Autodesk Inventor part; units mm, degrees
ref_plane "РабПлоскость7" through (-34.5, 0, 0) normal (-1, 0, 0) x (0, 0, 1)
ref_plane "YZ Plane" through (0, 0, 0) normal (1, 0, 0) x (0, 1, 0)
ref_plane "XZ Plane" through (0, 0, 0) normal (0, 1, 0) x (-1, 0, 0)
sketch "Эскиз1" plane through (0, 0, 0) normal (0, 1, 0) x (-1, 0, 0)
  line L0 (0, 0) -> (69, 0)
  line L1 (69, 0) -> (69, -52)
  line L2 (69, -52) -> (0, -52)
  line L3 (0, -52) -> (0, 0)
  line L4 (0, -26) -> (32, -26)
  line L5 (64, -10) -> (0, -10)
  line L6 (0, -10) -> (0, -42)
  line L7 (0, -42) -> (64, -42)
  line L8 (64, -42) -> (64, -10)
  line L9 (64, -10) -> (0, -42) construction
  line L10 (0, -10) -> (64, -42) construction
  line L11 (0, -10) -> (2, -10)
  point P0 (0, -10)
  dimension "d0" = 69
  dimension "d224" = 10
  dimension "d225" = 5
  dimension "d226" = 32
extrude "Выдавливание1" add sketch "Эскиз1" along normal blind 15 contours L0 L1 L2 L3 L7 L8 L5
sketch "Эскиз2" plane through (0, 15, 0) normal (0, 1, 0) x (1, 0, 0)
  line L0 (-8.5, 3.5) -> (-60.5, 3.5)
  line L1 (-60.5, 3.5) -> (-60.5, 48.5)
  line L2 (-60.5, 48.5) -> (-8.5, 48.5)
  line L3 (-8.5, 48.5) -> (-8.5, 3.5)
  line L4 (-8.5, 3.5) -> (-60.5, 48.5) construction
  line L5 (-60.5, 3.5) -> (-8.5, 48.5) construction
  line L6 (0, 0) -> (0, 10)
  line L7 (-69, 52) -> (-69, 0)
  line L8 (0, 52) -> (-69, 52) construction
  line L9 (0, 10) -> (0, 42) construction
  line L10 (-69, 26) -> (0, 26) construction
  point P0 (-34.5, 26)
  point P1 (-34.5, 26)
  point P2 (-60.5, 26)
  point P3 (-34.5, 26)
  dimension "d227" = 52
  dimension "d228" = 45
extrude "Выдавливание2" cut sketch "Эскиз2" against normal blind 3.5
sketch "Эскиз3" plane through (0, 11.5, 0) normal (0, 1, 0) x (1, 0, 0)
  circle A0 centre (-57.5, 45.5) radius 3
  circle A1 centre (-11.5, 45.5) radius 3
  line L0 (-60.5, 48.5) -> (-8.5, 48.5)
  line L1 (-8.5, 48.5) -> (-8.5, 42)
  line L2 (-8.5, 42) -> (-60.5, 42)
  line L3 (-60.5, 42) -> (-60.5, 48.5)
  line L4 (-60.5, 10) -> (-8.5, 10)
  line L5 (-8.5, 42) -> (-60.5, 42)
  line L6 (-8.5, 48.5) -> (-8.5, 42)
  line L7 (-60.5, 48.5) -> (-8.5, 48.5)
  line L8 (-60.5, 42) -> (-60.5, 48.5)
  line L9 (-60.5, 3.5) -> (-60.5, 10)
  line L10 (-8.5, 3.5) -> (-60.5, 3.5)
  line L11 (-8.5, 10) -> (-8.5, 3.5)
  line L12 (0, 10) -> (-64, 10)
  line L13 (-8.5, 3.5) -> (-60.5, 3.5)
  line L14 (-32, 3.5) -> (-37, 3.5)
  line L15 (-37, 3.5) -> (-37, 5.5)
  line L16 (-37, 5.5) -> (-32, 5.5)
  line L17 (-32, 5.5) -> (-32, 3.5)
  line L18 (-8.5, 3.5) -> (-60.5, 3.5)
  point P0 (-38, 39.1)
  point P1 (-60.5, 45.5)
  point P2 (-8.3, 39.1)
  point P3 (-5.8, 45.225)
  point P4 (-57.5, 48.5)
  point P5 (-11.5, 48.5)
  point P6 (-8.5, 42.24)
  point P7 (-8.5, 45.5)
  point P8 (-34.5, 3.5)
  dimension "d236" = 3
  dimension "d237" = 3
  dimension "d238" = 3
  dimension "d239" = 3
  dimension "d240" = 6
  dimension "d241" = 6
  dimension "d304" = 2
  dimension "d305" = 5
extrude "Выдавливание5" add sketch "Эскиз3" along normal blind 3 contours A0 | A0 L3 L0 | L0 L1 A1 | A1 | L15 L16 L17 L10
sketch "Эскиз4" plane through (-71.3, 14.5, -19.65) normal (0, 1, 0) x (0, 0, -1)
  arc A0 (25.85, -10.8) -> (28.85, -13.8) centre (25.85, -13.8) ccw
  arc A1 (28.85, -59.8) -> (25.85, -62.8) centre (25.85, -59.8) ccw
hole "Отверстие1" at (-57.5, 14.5, -45.5) at (-11.5, 14.5, -45.5) direction (0, -1, 0) diameter 3 depth 5
sketch "Эскиз32" plane through (0, 11.5, 0) normal (0, 1, 0) x (1, 0, 0)
  line L0 (-64, 10) -> (-64, 42)
  line L1 (-64, 47.775) -> (-43.5, 47.775)
  line L2 (-8.5, 3.5) -> (-60.5, 3.5)
  line L3 (-8.5, 10) -> (-8.5, 3.5)
  line L4 (-60.5, 48.5) -> (-8.5, 48.5)
  line L5 (-8.5, 48.5) -> (-8.5, 42)
  point P0 (0, 0)
  point P1 (-17.6, 6.862)
  point P2 (-5.3, 5.3)
  point P3 (-8.3, 2.3)
  point P4 (-64, 4.225)
  point P5 (-17.6, 45.087)
  dimension "d261" = 3.362
  dimension "d263" = 9.1
  dimension "d296" = 3.413
  dimension "d297" = 9.1
hole "Отверстие5" at (-17.6, 11.5, -6.862) at (-17.6, 11.5, -45.087) direction (0, -1, 0) diameter 3.2 end through all countersink diameter 6 countersink angle 90
sketch "Эскиз12" plane through (0, 15, 0) normal (0, -1, 0) x (1, 0, 0)
  line L0 (-60.5, -48.5) -> (-8.5, -48.5)
  line L1 (0, -52) -> (-69, -52)
  line L2 (-35.9, -52) -> (-33.1, -52) construction
  line L3 (-35.9, -53) -> (-33.1, -53)
  line L4 (-33.1, -51) -> (-35.9, -51)
  arc A0 (-35.9, -51) -> (-35.9, -53) centre (-35.9, -52) ccw
  arc A1 (-33.1, -53) -> (-33.1, -51) centre (-33.1, -52) ccw
  point P0 (-34.5, -52)
  dimension "d302" = 1.4
  dimension "d303" = 2
extrude "Выдавливание11" cut sketch "Эскиз12" along normal through all
sketch "Эскиз34" plane through (0, 15, 0) normal (0, 1, 0) x (1, 0, 0)
  line L0 (-5.35, 7.9) -> (-3.15, 7.9)
  line L1 (-3.15, 7.9) -> (-3.15, 10)
  line L2 (-3.15, 10) -> (-5.35, 10)
  line L3 (-5.35, 10) -> (-5.35, 7.9)
  line L4 (0, 10) -> (-8.5, 10)
  line L5 (-5.35, 42) -> (-3.15, 42)
  line L6 (-3.15, 42) -> (-3.15, 44.1)
  line L7 (-3.15, 44.1) -> (-5.35, 44.1)
  line L8 (-5.35, 44.1) -> (-5.35, 42)
  line L9 (-8.5, 42) -> (0, 42)
  point P0 (0, 0)
  point P1 (-4.25, 10)
  point P2 (-4.25, 42)
  dimension "d278" = 2.2
  dimension "d279" = 2.1
extrude "Выдавливание27" cut sketch "Эскиз34" against normal through all
sketch "Эскиз36" plane through (0, 0, 0) normal (0, -1, 0) x (1, 0, 0)
  line L0 (-64, -10) -> (-64, 0)
  line L1 (-69, 0) -> (0, 0)
  line L2 (-67, -9) -> (-42, -9)
  line L3 (-42, -9) -> (-42, -1)
  line L4 (-42, -1) -> (-67, -1)
  line L5 (-67, -1) -> (-67, -9)
  line L6 (-69, -52) -> (-69, 0)
  point P0 (-67, -5)
  point P1 (-64, -5)
  dimension "d285" = 2
  dimension "d286" = 8
  dimension "d287" = 25
extrude "Выдавливание29" cut sketch "Эскиз36" against normal blind 13.5
sketch "Эскиз37" plane through (-69, 0, -52) normal (-1, 0, 0) x (0, 0, 1)
  line L0 (43, 0) -> (51, 0)
  line L1 (43, 0) -> (43, 13.5)
  line L2 (43, 13.5) -> (51, 13.5)
  line L3 (51, 0) -> (51, 13.5)
  line L4 (43, 0) -> (43, 13.5) construction
  line L5 (43, 6.75) -> (51, 6.75) construction
  line L6 (51, 0) -> (51, 13.5) construction
  circle A0 centre (47, 6.75) radius 3.25
  point P0 (52, 0)
  dimension "d290" = 6.5
extrude "Выдавливание30" cut sketch "Эскиз37" against normal up to surface (2 mm away) contours A0
sketch "Эскиз38" plane through (0, 15, 0) normal (0, 1, 0) x (1, 0, 0)
  line L0 (-42, 3.5) -> (-45.5, 3.5)
  line L1 (-45.5, 3.5) -> (-45.5, 2)
  line L2 (-45.5, 2) -> (-42, 2)
  line L3 (-42, 2) -> (-42, 3.5)
  line L4 (-69, 0) -> (0, 0)
  line L5 (-42, 9) -> (-42, 3.5)
  dimension "d293" = 3.5
  dimension "d301" = 1.5
extrude "Выдавливание31" cut sketch "Эскиз38" against normal up to surface (1.5 mm away)
sketch "Эскиз30" plane through (0, 0, 0) normal (0, -1, 0) x (1, 0, 0)
  line L0 (-69, -39.85) -> (-67, -39.85)
  line L1 (-67, -39.85) -> (-67, -12.15)
  line L2 (-67, -12.15) -> (-69, -12.15)
  line L3 (-69, -12.15) -> (-69, -39.85)
  line L4 (-69, -52) -> (-69, 0)
  line L5 (-67, -39.85) -> (-68.1, -39.85)
  line L6 (-68.1, -39.85) -> (-68.1, -40.85)
  line L7 (-68.1, -40.85) -> (-67, -40.85)
  line L8 (-67, -40.85) -> (-67, -39.85)
  line L9 (-67, -12.15) -> (-68.5, -12.15)
  line L10 (-68.5, -12.15) -> (-68.5, -11.15)
  line L11 (-68.5, -11.15) -> (-67, -11.15)
  line L12 (-67, -11.15) -> (-67, -12.15)
  point P0 (0, 0)
  point P1 (-69, -26)
  point P2 (-68.5, -12.15)
  point P3 (-68.1, -39.85)
  dimension "d216" = 27.7
  dimension "d217" = 2
  dimension "d218" = 1.1
  dimension "d219" = 1
  dimension "d220" = 1.5
  dimension "d221" = 1
extrude "Выдавливание24" cut sketch "Эскиз30" against normal blind 13.1
chamfer "Фаска7" distance 4 angle 45 2 edges at (0, 7.5, -52) (-69, 7.5, -52)
sketch "Эскиз39" plane through (0, 15, 0) normal (0, 1, 0) x (1, 0, 0)
  line L0 (-69, 48) -> (-69, 0) construction
  line L1 (-69, 48) -> (-69, 73.55) construction
  line L2 (-69, 73.55) -> (-73.55, 73.55) construction
  line L3 (-73.55, 73.55) -> (-64.1507, 51.55) construction
  line L4 (-64.1507, 51.55) -> (-62.6872, 48.1245) construction
  circle A0 centre (-73.55, 73.55) radius 27.6488
  point P0 (0, 0)
  dimension "d316" = 25.55
  dimension "d317" = 4.55
  dimension "d319" = 22
  dimension "d320" = 3.725
  dimension "d321" = 23.134
extrude "Выдавливание32" cut sketch "Эскиз39" against normal blind 1.2
ref_plane "РабПлоскость7" through (-34.5, 0, 0) normal (-1, 0, 0) x (0, 0, 1)
mirror "Зеркальное отражение2" about plane through (-34.5, 0, 0) normal (-1, 0, 0) of "Выдавливание32"
properties part number "Стойка под электроннику"
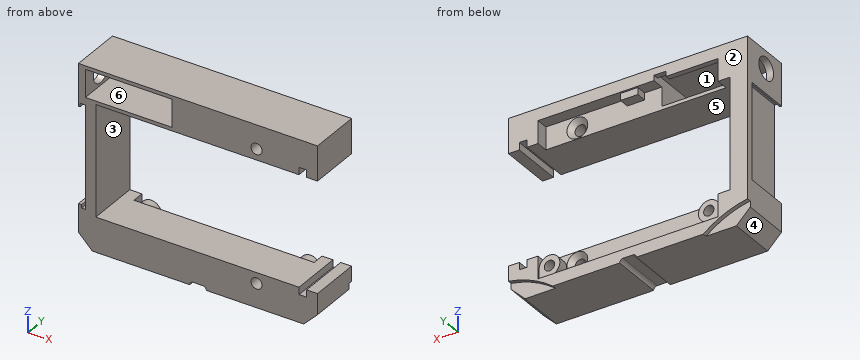
Model file for the job. Use its own axes, mm. Face numbers are marked on the shaded views. A direction names the side the tool comes from. Coordinates: 2 decimals unless noted, no trailing zeros. Order: outer loops, then holes, each group sorted by start corner. A loop starts at its lowest first (then second) coordinate and runs counter-clockwise, first axis right, second up. Notation, with made-up numbers: (87, 0.5) -> (118, 0.5) arc R7 cw to (118, 13.5) -> close; hole circle Ø11 at (29.5, -20.75). An arc over 180 degrees is marked (long way). Return JSON: item names as keys, results as strings. Group by question number.
Item 1: Saw through at B-B on z = -35.5. Write the cut outline in (x, y).
Item 2: Saw through at A-A on x = -17.6. Write the cut outline in (y, z), then the cut area to 3 significant figures.
Item 3: Tool access for the marked faces 4, 5 and 6: list every direction of +Z, -Z, +X, -X, +Y, -Y with a clear straight run to the whole face (end or side of a thin tool).
Item 4: Flat gauge pins, fed straight in: P1, Ø2, axis at y = 11, z = -15, coming from the -X side; P2, Ø8, axis at x = -36.5, y = 10.5, coming from the -Z side; P3, Ø0.5, axis at y = 5.5, z = -40.5, coming from the +X side; P4, Ø10, axis at x = -21.5, z = -12, coming from the +Y side. Where does each tip first touch, or does it go through?
Item 5: Saw through at C-C on x = -62.5. Write the cut outline in (y, z), then the cut area to 3 significant figures.
Item 6: Pull direction X, two halves, no side cores. Call the marked faces 1, 2 and 3: pulls with the +X half, pulls with the -X half, needs draft (parallel to the pull), parting line crosses it, or undercut.
Item 7: Saw through at D-D on y = 8.5. State how many separate pieces and enclosed holes the cut face has, then the cut area to 3 significant figures.
Item 8: Wall check: line 1 along Z through (x, y) = (-17.6, 5); line 2 along Z through (x, y) = (-52, 10); line 3 along Z through (x, y) = (-37.5, 1.5). Give the ranges that are in metal, low to high. Write a range as [from, to].
Values found:
{
 "1": {"outline": "(-69, 13.1) -> (-67, 13.1) -> (-67, 0) -> (-64, 0) -> (-64, 15) -> (-69, 15) -> close"},
 "2": {"outline": "(0, -52) -> (15, -52) -> (15, -48.5) -> (11.5, -48.5) -> (11.5, -48.09) -> (10.1, -46.69) -> (0, -46.69) -> close; (0, -43.49) -> (10.1, -43.49) -> (11.5, -42.09) -> (11.5, -42) -> (0, -42) -> close; (0, -10) -> (11.5, -10) -> (11.5, -9.86) -> (10.1, -8.46) -> (0, -8.46) -> close; (0, -5.26) -> (10.1, -5.26) -> (11.5, -3.86) -> (11.5, -3.5) -> (15, -3.5) -> (15, 0) -> (0, 0) -> close", "area": "177 mm2"},
 "3": {"face 4": "-Z, -X, +Y, -Y", "face 5": "+X, +Y, -Y", "face 6": "-Y"},
 "4": {"P1": "stops at x = -67", "P2": "stops at z = -52", "P3": "stops at x = -64", "P4": "stops at y = 11.5"},
 "5": {"outline": "(0, -52) -> (13.8, -52) -> (13.8, -48.21) -> (15, -48.21) -> (15, -42) -> (0, -42) -> close; (0, -10) -> (15, -10) -> (15, 0) -> (0, 0) -> (0, -1) -> (13.5, -1) -> (13.5, -9) -> (0, -9) -> close", "area": "187 mm2"},
 "6": {"face 1": "undercut", "face 2": "needs draft", "face 3": "pulls with the +X half"},
 "7": {"separate pieces": "1", "enclosed holes": "2", "area": "1,230 mm2"},
 "8": {"line 1": "z = [-52, -46.69], [-43.49, -42], [-10, -8.46], [-5.26, 0]", "line 2": "z = [-52, -42], [-10, -9], [-1, 0]", "line 3": "z = [-52, -42], [-10, 0]"}
}
